Could you check a few things on this model? Use its own coordinates, in mm. Round coordinates to 2 decimals unless told otherwise and drop trailing zeros. Loops run counter-clockwise (first coordinate to the right, second up) from the corner with the lowest first, then second, coordinate; pieces in that order, holes last. Notation, with made-up numbers: M -39.5,-37.5 L -28.5,-37.5 A21 ccw -28.5,-24.5 Z; hole C 33,55 d1. An arc over 180 degrees is marked long. One line per item, written item: value. Start each with the question number.
Q1. Imagine slicing it at C-C (x = 0). Please give me the cut outline in (y, z).
Q2. Imagine slicing it at B-B (z = 20). Please give me the cut outline in (x, y), then the cut area to 3 significant figures.
Q3. Please list where these lines run through material, in increasing order: line 1 along Y through (x, z) = (0, 10.25); line 2 along X through (y, z) = (-0.5, 15) (3 decimals); line 3 along Y through (x, z) = (7, 23.5).
Q4. Imagine slicing it at A-A (y = 70). Please give me the cut outline in (x, z).
Q5. I'm going to push flat-ended pins straight in: pin 1 Ø2 at (x, z) = (-12.5, 26) entering from -Y; pin 2 Ø10 at (x, z) = (14.5, 20) entering from -Y; pin 3 Ø10 at (x, z) = (5.5, 4) entering from -Y (3 decimals). Where does each tip first touch, or does it pass through?
from build123d import *

# Parameters (mm, degrees)
SKETCH1_R           = 15
BOSS_EXTRUDE1_DEPTH = 30


with BuildPart() as part:
    # Sketch1 → Boss-Extrude1 (new body)
    with BuildSketch(Plane.XY):
        with BuildLine():
            Line((-25, 0), (-25, 440))
            ThreePointArc((-25, 440), (0, 465), (25, 440))
            Line((25, 440), (25, 0))
            ThreePointArc((25, 0), (0, -25), (-25, 0))
        make_face()
        with Locations((0, 440)):
            Circle(SKETCH1_R, mode=Mode.SUBTRACT)
        with Locations((0, 308)):
            Circle(SKETCH1_R, mode=Mode.SUBTRACT)
        with Locations((0, 70)):
            Circle(SKETCH1_R, mode=Mode.SUBTRACT)
        Circle(SKETCH1_R, mode=Mode.SUBTRACT)
    extrude(amount=BOSS_EXTRUDE1_DEPTH)


solid = part.part
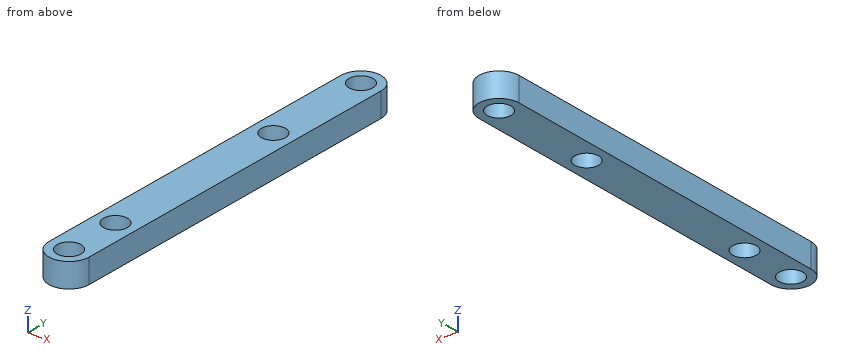
Report:
1. outline: M -25,0 L -15,0 L -15,30 L -25,30 Z; M 15,0 L 55,0 L 55,30 L 15,30 Z; M 85,0 L 293,0 L 293,30 L 85,30 Z; M 323,0 L 425,0 L 425,30 L 323,30 Z; M 455,0 L 465,0 L 465,30 L 455,30 Z
2. outline: M -25,0 A25 ccw 25,0 L 25,440 A25 ccw -25,440 Z; hole C 0,0 d30; hole C 0,70 d30; hole C 0,308 d30; hole C 0,440 d30
2. area: 21,100 mm²
3. line 1: y = -25 to -15, 15 to 55, 85 to 293, 323 to 425, 455 to 465
3. line 2: x = -24.995 to -14.992, 14.992 to 24.995
3. line 3: y = -24 to -13.27, 13.27 to 56.73, 83.27 to 294.73, 321.27 to 426.73, 453.27 to 464
4. outline: M -25,0 L -15,0 L -15,30 L -25,30 Z; M 15,0 L 25,0 L 25,30 L 15,30 Z
5. pin 1: stops at y = -22.2
5. pin 2: stops at y = -23.12
5. pin 3: stops at y = -24.995
